from build123d import *

# Parameters (mm, degrees)
CUT_EXTRUDE1_DEPTH      = 126.287668986
CUT_EXTRUDE1_DEPTH_BACK = 126.287668986
SKETCH3_W               = 4.7
SKETCH3_H               = 4.75
CUT_EXTRUDE2_DEPTH      = 126.287668986
CUT_EXTRUDE2_DEPTH_BACK = 126.287668986
SKETCH4_W               = 184.7
SKETCH4_H               = 3
CUT_EXTRUDE4_DEPTH      = 226.159943152
CUT_EXTRUDE4_DEPTH_BACK = 226.159943152
SKETCH5_W               = 15.463728056
SKETCH5_H               = 5.091329687
SKETCH5_H_2             = 5.301676888


with BuildPart() as part:
    # Sketch1 → Revolve1 (revolve)
    with BuildSketch(Plane(origin=(0, 0, 0), x_dir=(1, 0, 0), z_dir=(0, 1, 0)), mode=Mode.PRIVATE) as revolve1_sk:
        Polygon((-125, 0), (-125, 3.5), (-120, 3.5), (-116.802652106, 4), (78, 4), (80, 6), (100, 6), (100, 0), align=None)
    revolve(revolve1_sk.sketch.rotate(Axis((-125, 0, 0), (1, 0, 0)), 180), axis=Axis((-125, 0, 0), (1, 0, 0)))

    # Sketch3 → Cut-Extrude1 (cut, two sides: drawn at the far end of the back side and taken through both)
    with BuildSketch(Plane(origin=(0, 0, 0), x_dir=(1, 0, 0), z_dir=(0, 1, 0)).offset(-CUT_EXTRUDE1_DEPTH_BACK)):
        with Locations((-112, 1.625)):
            Rectangle(SKETCH3_W, SKETCH3_H)
        with Locations((-102, 1.625)):
            Rectangle(SKETCH3_W, SKETCH3_H)
        with Locations((-92, 1.625)):
            Rectangle(SKETCH3_W, SKETCH3_H)
        with Locations((-82, 1.625)):
            Rectangle(SKETCH3_W, SKETCH3_H)
        with Locations((-72, 1.625)):
            Rectangle(SKETCH3_W, SKETCH3_H)
        with Locations((-62, 1.625)):
            Rectangle(SKETCH3_W, SKETCH3_H)
        with Locations((-52, 1.625)):
            Rectangle(SKETCH3_W, SKETCH3_H)
        with Locations((-42, 1.625)):
            Rectangle(SKETCH3_W, SKETCH3_H)
        with Locations((-32, 1.625)):
            Rectangle(SKETCH3_W, SKETCH3_H)
        with Locations((-22, 1.625)):
            Rectangle(SKETCH3_W, SKETCH3_H)
        with Locations((-12, 1.625)):
            Rectangle(SKETCH3_W, SKETCH3_H)
        with Locations((-2, 1.625)):
            Rectangle(SKETCH3_W, SKETCH3_H)
        with Locations((8, 1.625)):
            Rectangle(SKETCH3_W, SKETCH3_H)
        with Locations((18, 1.625)):
            Rectangle(SKETCH3_W, SKETCH3_H)
        with Locations((28, 1.625)):
            Rectangle(SKETCH3_W, SKETCH3_H)
        with Locations((38, 1.625)):
            Rectangle(SKETCH3_W, SKETCH3_H)
        with Locations((48, 1.625)):
            Rectangle(SKETCH3_W, SKETCH3_H)
        with Locations((58, 1.625)):
            Rectangle(SKETCH3_W, SKETCH3_H)
        with Locations((68, 1.625)):
            Rectangle(SKETCH3_W, SKETCH3_H)
    extrude(amount=CUT_EXTRUDE1_DEPTH + CUT_EXTRUDE1_DEPTH_BACK, mode=Mode.SUBTRACT)

    # Sketch4 → Cut-Extrude2 (cut, two sides: drawn at the far end of the back side and taken through both)
    with BuildSketch(Plane(origin=(0, 0, 0), x_dir=(1, 0, 0), z_dir=(0, 1, 0)).offset(-CUT_EXTRUDE2_DEPTH_BACK)):
        with Locations((-22, 2.5)):
            Rectangle(SKETCH4_W, SKETCH4_H)
    extrude(amount=CUT_EXTRUDE2_DEPTH + CUT_EXTRUDE2_DEPTH_BACK, mode=Mode.SUBTRACT)

    # Sketch5 → Cut-Extrude4 (cut, two sides: drawn at the far end of the back side and taken through both)
    with BuildSketch(Plane.ZY.offset(125).offset(-CUT_EXTRUDE4_DEPTH_BACK)):
        with Locations((0.057906168, -4.545664844)):
            Rectangle(SKETCH5_W, SKETCH5_H)
        with Locations((0.057906168, 4.650838444)):
            Rectangle(SKETCH5_W, SKETCH5_H_2)
    extrude(amount=CUT_EXTRUDE4_DEPTH + CUT_EXTRUDE4_DEPTH_BACK, mode=Mode.SUBTRACT)


solid = part.part
Verification items for the finished model (mm, model axes). A direction names the side the tool comes from. Coordinates: 2 decimals unless noted, no trailing zeros. Write each loop counter-clockwise with the first axis right and the second up, starting at its lowest first coordinate (ties: lowest second). Pieces come first, ordered by that corner, then holes. Notation, with made-up numbers: (10.5, -18) -> (22.5, -18) arc R9 ccw to (22.5, -7) -> close; hole circle Ø6 at (-39, 27). An arc over 180 degrees is marked (long way). One line per item, written item: value. Start each with the question number.
Q1. Access from +Z, -Z, +X, -X, +Y, -Y to the whole of each face (thin tool, end or side, straight path). Record for faces 3 (the flat face through (8, 0, 0.75)), 4 (the cylindrical face through (-18, 0, 4)), 5 (the cylindrical face through (90, 0, -6)).
Q2. Cross-section at A-A on x = 83.5. Enter the section's corners in (y, z).
Q3. Go/stop test with flat-tipped pins: P1, Ø2, axis at x = -53, y = 1, coming from the +Z side; P2, Ø1.2, axis at x = -43, y = -0.5, coming from the -Z side. Record where each tip stops, or that it passes through.
Q4. Thickness scan on L1, parallel to X at y = 1.4, z = -1.75; L2, parallel to Z at x = -29.5, y = 0.5; L3, parallel to Z at x = -6, y = 1.8. Record the ranges inside material, lowest first. Write a range as from..to.
Q5. Cross-section at B-B on x = 38. Enter the section's corners in (y, z), and give its area (3 significant figures).
Q6. Mould release check, pull along X, two halves, no side actions. Record for faces 1 (the flat face through (68, 0, 0.75)), 2 (the cylindrical face through (-122.5, 0, -3.5)): pulls with the +X half, pulls with the -X half, needs draft (parallel to the pull), parting line crosses it, or undercut.
Checked values:
1. face 3: -Z, +Y, -Y
1. face 4: +Z, -X
1. face 5: -Z, +X, -X
2. outline: (-2, -5.66) arc R6 ccw to (2, -5.66) -> (2, 5.66) arc R6 ccw to (-2, 5.66) -> close
3. P1: stops at z = 4
3. P2: stops at z = 0.75
4. L1: x = -125..-114.35, 70.35..100
4. L2: z = -1..3.97
4. L3: z = -1..3.57
5. outline: (-2, 0.75) -> (2, 0.75) -> (2, 3.46) arc R4 ccw to (-2, 3.46) -> close
5. area: 12.3 mm²
6. face 1: undercut
6. face 2: needs draft
